Build history of the part. All positions in model axes, mm. A direction names the side the tool comes from. Coordinates: 2 decimals unless noted, no trailing zeros. Loops run counter-clockwise (first coordinate to the right, second up) from the corner with the lowest first, then second, coordinate; pieces in that order, holes last. Notation, with made-up numbers: (-21.5, 50) - (-5.5, 50) arc R11 cw to (-5.5, 64) - close; hole circle Ø2 at (-7.75, 73). An arc over 180 degrees is marked (long way). One line per item, written item: value.
```python
from build123d import *

# Parameters (mm, degrees)
SKETCH1_W           = 400
SKETCH1_H           = 30
BOSS_EXTRUDE1_DEPTH = 50
SKETCH2_W           = 400
SKETCH2_H           = 10
BOSS_EXTRUDE2_DEPTH = 310
CUT_EXTRUDE1_DEPTH  = 400
LPATTERN1_COUNT     = 15
LPATTERN1_PITCH     = 20


with BuildPart() as part:
    # Sketch1 → Boss-Extrude1 (new body)
    with BuildSketch(Plane(origin=(0, 0, 0), x_dir=(1, 0, 0), z_dir=(0, 1, 0))):
        with Locations((200, 15)):
            Rectangle(SKETCH1_W, SKETCH1_H)
    extrude(amount=BOSS_EXTRUDE1_DEPTH)

    # Sketch2 → Boss-Extrude2 (add)
    with BuildSketch(Plane.XY):
        with Locations((200, 35)):
            Rectangle(SKETCH2_W, SKETCH2_H)
    extrude(amount=BOSS_EXTRUDE2_DEPTH)

    # Sketch3 → Cut-Extrude1 (cut)
    with BuildSketch(Plane.ZY):
        Polygon((0, 40), (9.867375243, 36.624338333), (18.617949732, 40), align=None)
        Polygon((13.283352971, 30), (19.738366334, 33.302751996), (26.012819883, 30), align=None)
    cut_extrude1 = extrude(amount=-CUT_EXTRUDE1_DEPTH, mode=Mode.SUBTRACT)

    # LPattern1: Cut-Extrude1 ×15
    with Locations(*[(0, 0, i * LPATTERN1_PITCH) for i in range(1, LPATTERN1_COUNT)]):
        add(cut_extrude1, mode=Mode.SUBTRACT)


solid = part.part
```
Item 1: Drop flat-ended pins along their axis: P1, Ø8, axis at x = 331, z = 127.5, coming from the -Y side; P2, Ø1.5, axis at x = 245.5, z = 239.5, coming from the +Y side; P3, Ø8, axis at x = 276.5, z = 173, coming from the +Y side. Give the stop position or say it passes through.
Check result:
P1: stops at y = 30
P2: stops at y = 40
P3: stops at y = 39.38
Item 2: Tool access for faces 1 (the face through (197, 0, -15)), 2 (the face through (197.2, 38.336, 4.865)): list every direction of +Z, -Z, +X, -X, +Y, -Y with a clear straight run to the whole face (end or side of a thin tool).
Check result:
face 1: +Z, -Z, +X, -X, -Y
face 2: +X, -X, +Y
Item 3: Probe probe 1 along Z at (x, y) = (161.5, 29); probe 2 along Y at (x, z) = (73, 55); probe 3 along Y at (x, z) = (312.5, 138.5). List the from-to ranges inside material, lowest first. Write a range as from..to.
Check result:
probe 1: z = -30..0
probe 2: y = 30.88..38.6
probe 3: y = 32.67..39.95
Item 4: Pull direction Z, two halves, no side cores. Call faces 3 (the face through (197.2, 38.336, 244.865)), 4 (the face through (197, 50, -15)), 5 (the face through (197, 15, 0)): released by +Z, released by -Z, zero draft, split by the parting line, or undercut.
Check result:
face 3: undercut
face 4: zero draft
face 5: released by +Z
Item 5: Cut at A-A, the plane y = 22.5. Write the cut outline in (x, z).
Check result:
outline: (0, -30) - (400, -30) - (400, 0) - (0, 0) - close
